Here's how the part is built. I have some questions about the finished solid (model axes, mm). A direction names the side the tool comes from. Round coordinates to 2 decimals unless told otherwise and drop trailing zeros. Order: outer loops, then holes, each group sorted by start corner. A loop starts at its lowest first (then second) coordinate and runs counter-clockwise, first axis right, second up. Notation, with made-up numbers: (35, -6.75) - (81, -6.75) arc R23 cw to (81, 22.25) - close; hole circle Ø10 at (22, 40.5). An arc over 180 degrees is marked (long way). Answer as a JSON object with one key per item and string values.
```python
from build123d import *
from OCP.BRepFilletAPI import BRepFilletAPI_MakeChamfer

# Parameters (mm, degrees)
EXTRUDE_1_DEPTH     = 48
SKETCH_3_R          = 2.4
CUT_EXTRUDE_2_DEPTH = 89.328704281
CUT_EXTRUDE_3_REACH = 90.108
CHAMFER_1_SIZE      = 0.2
FILLET_1_R          = 7
CUT_EXTRUDE_4_DEPTH = 88.011263639
FILLET_2_R          = 4
RIB_START           = -3.5
RIB_2_DEPTH         = 3.5
CHAMFER_2_SIZE      = 0.8
CHAMFER_2_SIZE2     = 0.291176187
CHAMFER_3_SIZE      = 0.8
CHAMFER_3_SIZE2     = 0.291176187
CHAMFER_4_SIZE      = 2
SKETCH_21_W         = 8.512208597
SKETCH_21_H         = 13.260826712
CUT_EXTRUDE_5_DEPTH = 88.011263639
SKETCH_22_W         = 4
SKETCH_22_H         = 5.7
EXTRUDE_4_DEPTH     = 48
SKETCH_23_W         = 3
SKETCH_23_H         = 23
EXTRUDE_5_DEPTH     = 8
SKETCH_25_R         = 2.4
CUT_EXTRUDE_6_DEPTH = 85.112781431


# Read off the part's stored shape, not the designer's step: 筋2
with BuildPart() as part:
    # 草图1 → 凸台-拉伸1 (new body)
    with BuildSketch(Plane.XY):
        Polygon((-10, -10), (-10, -13), (71.4, -13), (71.4, -9), (13, -9), (13, 10), (10, 10), (10, 2.95), (8, 2.95), (8, 4.75), (6.8, 4.75), (6, 3.95), (6, -3.95), (6.8, -4.75), (8, -4.75), (8, -2.95), (10, -2.95), (10, -10), align=None)
    extrude(amount=EXTRUDE_1_DEPTH)

    # 草图3 → 切除-拉伸2 (cut, through all)
    with BuildSketch(Plane(origin=(0, -10, 0), x_dir=(1, 0, 0), z_dir=(0, 1, 0))):
        with Locations(Location((0, -24, 0), (0, 0, 270))):
            Circle(SKETCH_3_R)
    extrude(amount=-CUT_EXTRUDE_2_DEPTH, mode=Mode.SUBTRACT)

    # 草图4 → 切除-拉伸3 (cut, up to next)
    with BuildSketch(Plane(origin=(0, -9, 0), x_dir=(1, 0, 0), z_dir=(0, 1, 0)), mode=Mode.PRIVATE) as cut_extrude_3_sk1:
        with BuildLine():
            Line((18.5, -6.8), (65.9, -6.8))
            ThreePointArc((65.9, -6.8), (67.6, -8.5), (65.9, -10.2))
            Line((65.9, -10.2), (18.5, -10.2))
            ThreePointArc((18.5, -10.2), (16.8, -8.5), (18.5, -6.8))
        make_face()
    cut_extrude_3_tool1 = extrude(cut_extrude_3_sk1.sketch, amount=-CUT_EXTRUDE_3_REACH, mode=Mode.PRIVATE) & part.part
    # 草图4 → 切除-拉伸3 (cut, up to next)
    with BuildSketch(Plane(origin=(0, -9, 0), x_dir=(1, 0, 0), z_dir=(0, 1, 0)), mode=Mode.PRIVATE) as cut_extrude_3_sk2:
        with BuildLine():
            Line((18.5, -37.8), (65.9, -37.8))
            ThreePointArc((65.9, -37.8), (67.6, -39.5), (65.9, -41.2))
            Line((65.9, -41.2), (18.5, -41.2))
            ThreePointArc((18.5, -41.2), (16.8, -39.5), (18.5, -37.8))
        make_face()
    cut_extrude_3_tool2 = extrude(cut_extrude_3_sk2.sketch, amount=-CUT_EXTRUDE_3_REACH, mode=Mode.PRIVATE) & part.part
    # 草图4 → 切除-拉伸3 (cut, up to next)
    with BuildSketch(Plane(origin=(0, -9, 0), x_dir=(1, 0, 0), z_dir=(0, 1, 0)), mode=Mode.PRIVATE) as cut_extrude_3_sk3:
        with BuildLine():
            Line((34, -12.5), (50.4, -12.5))
            ThreePointArc((50.4, -12.5), (61.9, -24), (50.4, -35.5))
            Line((50.4, -35.5), (34, -35.5))
            ThreePointArc((34, -35.5), (22.5, -24), (34, -12.5))
        make_face()
    cut_extrude_3_tool3 = extrude(cut_extrude_3_sk3.sketch, amount=-CUT_EXTRUDE_3_REACH, mode=Mode.PRIVATE) & part.part
    add(cut_extrude_3_tool1.solids().sort_by_distance((42.2, -9, 8.5))[0], mode=Mode.SUBTRACT)
    add(cut_extrude_3_tool2.solids().sort_by_distance((42.2, -9, 39.5))[0], mode=Mode.SUBTRACT)
    add(cut_extrude_3_tool3.solids().sort_by_distance((42.2, -9, 24))[0], mode=Mode.SUBTRACT)

    # 倒角1
    chamfer_1_edges = [part.edges().sort_by_distance(p)[0] for p in [
        (8, -2.95, 24),
        (8, -4.75, 24),
        (8, 4.75, 24),
        (8, 2.95, 24),
    ]]
    chamfer(chamfer_1_edges, length=CHAMFER_1_SIZE)

    # 圆角1
    fillet_1_edges = [part.edges().sort_by_distance(p)[0] for p in [
        (71.4, -11, 48),
        (71.4, -11, 0),
    ]]
    fillet(fillet_1_edges, radius=FILLET_1_R)

    # 草图11 → 切除-拉伸4 (cut, through all)
    with BuildSketch(Plane(origin=(0, 0, 0), x_dir=(-1, 0, 0), z_dir=(0, 0, -1))):
        Polygon((-10, -2.65), (-6, 0.706398525), (-6, -6.71507999), (-10, -6.71507999), align=None)
    extrude(amount=-CUT_EXTRUDE_4_DEPTH, mode=Mode.SUBTRACT)

    # 圆角2
    fillet_2_edges = [part.edges().sort_by_distance(p)[0] for p in [
        (6, 0.706398525, 24),
    ]]
    fillet(fillet_2_edges, radius=FILLET_2_R)

    # 筋2 outline → 筋2 (add)
    with BuildSketch(Plane.XY.offset(48).offset(RIB_START)):
        with BuildLine():
            Line((13, -9), (46, -9))
            Line((46, -9), (43, -6))
            Line((43, -6), (24.9, -6))
            ThreePointArc((24.9, -6), (18.606749647, -3.393250353), (16, 2.9))
            Line((16, 2.9), (16, 7))
            Line((16, 7), (13, 10))
            Line((13, 10), (13, -9))
        make_face()
    rib_2 = extrude(amount=RIB_2_DEPTH)

    # 镜向1: 筋2 across plane
    add(rib_2.mirror(Plane.XY.offset(24)))

    # 倒角2: one chamfer whose edges measure the first distance from different faces: ONE call of the kernel's chamfer builder (chamfer() names one face for all edges)
    chamfer_2_edges_1 = [part.edges().sort_by_distance(p)[0] for p in [
        (9.1, 2.95, 48),
    ]]
    chamfer_2_side_1 = [part.faces().sort_by_distance(p)[0] for p in [
        (9.1, 2.95, 24),
    ]]
    chamfer_2_edges_2 = [part.edges().sort_by_distance(p)[0] for p in [
        (8, 3.85, 48),
    ]]
    chamfer_2_side_2 = [part.faces().sort_by_distance(p)[0] for p in [
        (8, 3.85, 24),
    ]]
    chamfer_2_edges_3 = [part.edges().sort_by_distance(p)[0] for p in [
        (7.3, 4.75, 48),
    ]]
    chamfer_2_side_3 = [part.faces().sort_by_distance(p)[0] for p in [
        (7.3, 4.75, 24),
    ]]
    chamfer_2_edges_4 = [part.edges().sort_by_distance(p)[0] for p in [
        (7.9, 4.65, 48),
    ]]
    chamfer_2_side_4 = [part.faces().sort_by_distance(p)[0] for p in [
        (7.9, 4.65, 24),
    ]]
    chamfer_2_edges_5 = [part.edges().sort_by_distance(p)[0] for p in [
        (8.1, 3.05, 48),
    ]]
    chamfer_2_side_5 = [part.faces().sort_by_distance(p)[0] for p in [
        (8.1, 3.05, 24),
    ]]
    chamfer_2_edges_6 = [part.edges().sort_by_distance(p)[0] for p in [
        (8.714424781, -1.571274308, 48),
    ]]
    chamfer_2_side_6 = [part.faces().sort_by_distance(p)[0] for p in [
        (8.714424781, -1.571274308, 24),
    ]]
    chamfer_2_edges_7 = [part.edges().sort_by_distance(p)[0] for p in [
        (6.374768852, 0.88115611, 48),
    ]]
    chamfer_2_side_7 = [part.faces().sort_by_distance(p)[0] for p in [
        (6.374768852, 0.88115611, 24),
    ]]
    chamfer_2_edges_8 = [part.edges().sort_by_distance(p)[0] for p in [
        (6.4, 4.35, 48),
    ]]
    chamfer_2_side_8 = [part.faces().sort_by_distance(p)[0] for p in [
        (6.4, 4.35, 24),
    ]]
    chamfer_2_edges_9 = [part.edges().sort_by_distance(p)[0] for p in [
        (6, 3.260814579, 48),
    ]]
    chamfer_2_side_9 = [part.faces().sort_by_distance(p)[0] for p in [
        (6, 3.260814579, 24),
    ]]
    chamfer_2 = BRepFilletAPI_MakeChamfer(part.part.solid().wrapped)
    for e in chamfer_2_edges_1:
        chamfer_2.Add(CHAMFER_2_SIZE, CHAMFER_2_SIZE2, e.wrapped, chamfer_2_side_1[0].wrapped)  # the first distance lies on this face
    for e in chamfer_2_edges_2:
        chamfer_2.Add(CHAMFER_2_SIZE, CHAMFER_2_SIZE2, e.wrapped, chamfer_2_side_2[0].wrapped)  # the first distance lies on this face
    for e in chamfer_2_edges_3:
        chamfer_2.Add(CHAMFER_2_SIZE, CHAMFER_2_SIZE2, e.wrapped, chamfer_2_side_3[0].wrapped)  # the first distance lies on this face
    for e in chamfer_2_edges_4:
        chamfer_2.Add(CHAMFER_2_SIZE, CHAMFER_2_SIZE2, e.wrapped, chamfer_2_side_4[0].wrapped)  # the first distance lies on this face
    for e in chamfer_2_edges_5:
        chamfer_2.Add(CHAMFER_2_SIZE, CHAMFER_2_SIZE2, e.wrapped, chamfer_2_side_5[0].wrapped)  # the first distance lies on this face
    for e in chamfer_2_edges_6:
        chamfer_2.Add(CHAMFER_2_SIZE, CHAMFER_2_SIZE2, e.wrapped, chamfer_2_side_6[0].wrapped)  # the first distance lies on this face
    for e in chamfer_2_edges_7:
        chamfer_2.Add(CHAMFER_2_SIZE, CHAMFER_2_SIZE2, e.wrapped, chamfer_2_side_7[0].wrapped)  # the first distance lies on this face
    for e in chamfer_2_edges_8:
        chamfer_2.Add(CHAMFER_2_SIZE, CHAMFER_2_SIZE2, e.wrapped, chamfer_2_side_8[0].wrapped)  # the first distance lies on this face
    for e in chamfer_2_edges_9:
        chamfer_2.Add(CHAMFER_2_SIZE, CHAMFER_2_SIZE2, e.wrapped, chamfer_2_side_9[0].wrapped)  # the first distance lies on this face
    add(Compound.cast(chamfer_2.Shape()), mode=Mode.REPLACE)

    # 倒角3: one chamfer whose edges measure the first distance from different faces: ONE call of the kernel's chamfer builder (chamfer() names one face for all edges)
    chamfer_3_edges_1 = [part.edges().sort_by_distance(p)[0] for p in [
        (7.3, 4.75, 0),
    ]]
    chamfer_3_side_1 = [part.faces().sort_by_distance(p)[0] for p in [
        (7.3, 4.75, 23.6),
    ]]
    chamfer_3_edges_2 = [part.edges().sort_by_distance(p)[0] for p in [
        (8, 3.85, 0),
    ]]
    chamfer_3_side_2 = [part.faces().sort_by_distance(p)[0] for p in [
        (8, 3.85, 23.6),
    ]]
    chamfer_3_edges_3 = [part.edges().sort_by_distance(p)[0] for p in [
        (7.9, 4.65, 0),
    ]]
    chamfer_3_side_3 = [part.faces().sort_by_distance(p)[0] for p in [
        (7.9, 4.65, 23.6),
    ]]
    chamfer_3_edges_4 = [part.edges().sort_by_distance(p)[0] for p in [
        (8.1, 3.05, 0),
    ]]
    chamfer_3_side_4 = [part.faces().sort_by_distance(p)[0] for p in [
        (8.1, 3.05, 23.6),
    ]]
    chamfer_3_edges_5 = [part.edges().sort_by_distance(p)[0] for p in [
        (6, 3.260814579, 0),
    ]]
    chamfer_3_side_5 = [part.faces().sort_by_distance(p)[0] for p in [
        (6, 3.260814579, 23.6),
    ]]
    chamfer_3_edges_6 = [part.edges().sort_by_distance(p)[0] for p in [
        (6.4, 4.35, 0),
    ]]
    chamfer_3_side_6 = [part.faces().sort_by_distance(p)[0] for p in [
        (6.4, 4.35, 23.6),
    ]]
    chamfer_3_edges_7 = [part.edges().sort_by_distance(p)[0] for p in [
        (9.1, 2.95, 0),
    ]]
    chamfer_3_side_7 = [part.faces().sort_by_distance(p)[0] for p in [
        (9.1, 2.95, 23.6),
    ]]
    chamfer_3_edges_8 = [part.edges().sort_by_distance(p)[0] for p in [
        (8.714424781, -1.571274308, 0),
    ]]
    chamfer_3_side_8 = [part.faces().sort_by_distance(p)[0] for p in [
        (8.714424781, -1.571274308, 23.6),
    ]]
    chamfer_3_edges_9 = [part.edges().sort_by_distance(p)[0] for p in [
        (6.374768852, 0.88115611, 0),
    ]]
    chamfer_3_side_9 = [part.faces().sort_by_distance(p)[0] for p in [
        (6.374768852, 0.88115611, 23.6),
    ]]
    chamfer_3 = BRepFilletAPI_MakeChamfer(part.part.solid().wrapped)
    for e in chamfer_3_edges_1:
        chamfer_3.Add(CHAMFER_3_SIZE, CHAMFER_3_SIZE2, e.wrapped, chamfer_3_side_1[0].wrapped)  # the first distance lies on this face
    for e in chamfer_3_edges_2:
        chamfer_3.Add(CHAMFER_3_SIZE, CHAMFER_3_SIZE2, e.wrapped, chamfer_3_side_2[0].wrapped)  # the first distance lies on this face
    for e in chamfer_3_edges_3:
        chamfer_3.Add(CHAMFER_3_SIZE, CHAMFER_3_SIZE2, e.wrapped, chamfer_3_side_3[0].wrapped)  # the first distance lies on this face
    for e in chamfer_3_edges_4:
        chamfer_3.Add(CHAMFER_3_SIZE, CHAMFER_3_SIZE2, e.wrapped, chamfer_3_side_4[0].wrapped)  # the first distance lies on this face
    for e in chamfer_3_edges_5:
        chamfer_3.Add(CHAMFER_3_SIZE, CHAMFER_3_SIZE2, e.wrapped, chamfer_3_side_5[0].wrapped)  # the first distance lies on this face
    for e in chamfer_3_edges_6:
        chamfer_3.Add(CHAMFER_3_SIZE, CHAMFER_3_SIZE2, e.wrapped, chamfer_3_side_6[0].wrapped)  # the first distance lies on this face
    for e in chamfer_3_edges_7:
        chamfer_3.Add(CHAMFER_3_SIZE, CHAMFER_3_SIZE2, e.wrapped, chamfer_3_side_7[0].wrapped)  # the first distance lies on this face
    for e in chamfer_3_edges_8:
        chamfer_3.Add(CHAMFER_3_SIZE, CHAMFER_3_SIZE2, e.wrapped, chamfer_3_side_8[0].wrapped)  # the first distance lies on this face
    for e in chamfer_3_edges_9:
        chamfer_3.Add(CHAMFER_3_SIZE, CHAMFER_3_SIZE2, e.wrapped, chamfer_3_side_9[0].wrapped)  # the first distance lies on this face
    add(Compound.cast(chamfer_3.Shape()), mode=Mode.REPLACE)

    # 倒角4
    chamfer_4_edges = [part.edges().sort_by_distance(p)[0] for p in [
        (13, -9, 24),
    ]]
    chamfer(chamfer_4_edges, length=CHAMFER_4_SIZE)

    # 草图21 → 切除-拉伸5 (cut, through all)
    with BuildSketch(Plane.XY.offset(48)):
        with Locations((5.743895701, 1.572706777)):
            Rectangle(SKETCH_21_W, SKETCH_21_H)
    extrude(amount=-CUT_EXTRUDE_5_DEPTH, mode=Mode.SUBTRACT)

    # 草图22 → 凸台-拉伸4 (add)
    with BuildSketch(Plane.XY.offset(48)):
        with Locations((8, 0.25)):
            Rectangle(SKETCH_22_W, SKETCH_22_H)
    extrude(amount=-EXTRUDE_4_DEPTH)

    # 草图23 → 凸台-拉伸5 (add)
    with BuildSketch(Plane.XY.offset(48)):
        with Locations((11.5, -1.5)):
            Rectangle(SKETCH_23_W, SKETCH_23_H)
    extrude_5 = extrude(amount=EXTRUDE_5_DEPTH)

    # 草图25 → 切除-拉伸6 (cut, through all)
    with BuildSketch(Plane.ZY.offset(-10)):
        with Locations((52, 0)):
            Circle(SKETCH_25_R)
    cut_extrude_6 = extrude(amount=-CUT_EXTRUDE_6_DEPTH, mode=Mode.SUBTRACT)

    # 镜向2: 凸台-拉伸5, 切除-拉伸6 across plane
    add(extrude_5.mirror(Plane.XY.offset(24)))
    add(cut_extrude_6.mirror(Plane.XY.offset(24)), mode=Mode.SUBTRACT)


solid = part.part
```
1. Imagine slicing it at C-C (z = 24). List the corners of the cut face in (x, y) for me, plus the area to 3 significant figures.
Responses:
{"outline": "(-10, -13) - (-2.4, -13) - (-2.4, -10) - (-10, -10) - close; (2.4, -13) - (22.5, -13) - (22.5, -9) - (15, -9) - (13, -7) - (13, 10) - (10, 10) - (10, 3.1) - (6, 3.1) - (6, -2.6) - (10, -2.6) - (10, -10) - (2.4, -10) - close; (61.9, -13) - (71.4, -13) - (71.4, -9) - (61.9, -9) - close", "area": "215 mm2"}
2. For P1, Ø1, axis at y = 4.5, z = 46, coming from the +X side; P2, Ø2, axis at y = -6, z = 45, coming from the -X side; P3, Ø12, axis at x = 22.5, z = 13.5, coming from the +Y side, each with a flat end and sliding along its axis, tell me the tip position at first contact or that it passes through.
Responses:
{"P1": "x = 16", "P2": "x = 10", "P3": "y = -9"}
3. Imagine slicing it at B-B (x = 45). List the corners of the cut face in (y, z) for me, plus the area to 3 significant figures.
Responses:
{"outline": "(-13, 0) - (-8, 0) - (-8, 3.5) - (-9, 3.5) - (-9, 6.8) - (-13, 6.8) - close; (-13, 10.2) - (-9, 10.2) - (-9, 12.5) - (-13, 12.5) - close; (-13, 35.5) - (-9, 35.5) - (-9, 37.8) - (-13, 37.8) - close; (-13, 41.2) - (-9, 41.2) - (-9, 44.5) - (-8, 44.5) - (-8, 48) - (-13, 48) - close", "area": "79.8 mm2"}
4. Imagine slicing it at D-D (x = 0). List the corners of the cut face in (y, z) for me.
Responses:
{"outline": "(-13, 0) - (-10, 0) - (-10, 21.6) - (-13, 21.6) - close; (-13, 26.4) - (-10, 26.4) - (-10, 48) - (-13, 48) - close"}
5. Thinking about a two-plate mould opening in Z: for faces 4 (the face through (16.8, -11, 8.5)), 5 (the face through (31, -8, 48)), 6 (the face through (14, -8, 24)), 7 (the face through (21, -13, 24)), which applies, pulls with the +Z half, pulls with the -Z half, needs draft (parallel to the pull), parting line crosses it, or undercut?
Responses:
{"face 4": "undercut", "face 5": "pulls with the +Z half", "face 6": "undercut", "face 7": "needs draft"}
6. For faces 1 (the face through (16, 5, 46)), 2 (the face through (13, -2, -2)), 3 (the face through (43, -11, 41.2)), which set-ups out of +Z, -Z, +X, -X, +Y, -Y let a thin tool reach every point of the face, with its end or its side?
Responses:
{"face 1": "+Z, -Z, +X, +Y", "face 2": "-Z, +X, +Y, -Y", "face 3": "+Y, -Y"}
7. Imagine slicing it at A-A (z = 8.5). List the corners of the cut face in (x, y) for me.
Responses:
{"outline": "(-10, -13) - (16.8, -13) - (16.8, -9) - (15, -9) - (13, -7) - (13, 10) - (10, 10) - (10, 3.1) - (6, 3.1) - (6, -2.6) - (10, -2.6) - (10, -10) - (-10, -10) - close; (67.6, -13) - (71.4, -13) - (71.4, -9) - (67.6, -9) - close"}
8. If I drill on L1, parallel to X at y = -10.8, z = 24; L2, parallel to Z at x = 39.5, y = -10.25; L3, parallel to Y at x = 12, z = 52, over which ranges is the centre line in solid material (lowest first)? Write a range as [from, to].
Responses:
{"L1": "[-10, -2.4], [2.4, 22.5], [61.9, 71.4]", "L2": "[0, 6.8], [10.2, 12.5], [35.5, 37.8], [41.2, 48]", "L3": "[-13, -2.4], [2.4, 10]"}
